```python
from build123d import *

# Parameters (mm, degrees)
ESQUISSE1_W             = 16
ESQUISSE1_H             = 28.1
ESQUISSE1_R             = 1.725
BOSS_EXTRU_1_DEPTH      = 8.6
ESQUISSE2_W             = 16
ESQUISSE2_H             = 14.6
ENL_V_MAT_EXTRU_2_DEPTH = 7
ENL_V_MAT_EXTRU_5_DEPTH = 16
ENL_V_MAT_EXTRU_6_DEPTH = 7
ENL_V_START             = -2
ENL_V_MAT_EXTRU_9_DEPTH = 18


with BuildPart() as part:
    # Esquisse1 → Boss.-Extru.1 (new body)
    with BuildSketch(Plane.XY):
        with Locations((-5.445538763, -0.094706778)):
            Rectangle(ESQUISSE1_W, ESQUISSE1_H)
        with Locations(Location((-5.445538763, 10.955293222, 0), (0, 0, 180))):
            Circle(ESQUISSE1_R, mode=Mode.SUBTRACT)
        with Locations(Location((-5.445538763, -11.144706778, 0), (0, 0, 180))):
            Circle(ESQUISSE1_R, mode=Mode.SUBTRACT)
    extrude(amount=BOSS_EXTRU_1_DEPTH)

    # Esquisse2 → Enlèv. mat.-Extru.2 (cut)
    with BuildSketch(Plane(origin=(0, 0, 0), x_dir=(-1, 0, 0), z_dir=(0, 0, -1))):
        with Locations((5.445538763, -0.344706778)):
            Rectangle(ESQUISSE2_W, ESQUISSE2_H)
    extrude(amount=-ENL_V_MAT_EXTRU_2_DEPTH, mode=Mode.SUBTRACT)

    # Esquisse4 → Enlèv. mat.-Extru.5 (cut)
    with BuildSketch(Plane(origin=(0, 0, 0), x_dir=(-1, 0, 0), z_dir=(0, 0, -1))):
        Polygon((8.103346265, -14.144706778), (13.445538763, -14.144706778), (13.445538763, -8.673372576), (6.156041758, -14.144706778), align=None)
    extrude(amount=-ENL_V_MAT_EXTRU_5_DEPTH, mode=Mode.SUBTRACT)

    # Esquisse5 → Enlèv. mat.-Extru.6 (cut)
    with BuildSketch(Plane(origin=(0, 0, 0), x_dir=(-1, 0, 0), z_dir=(0, 0, -1))):
        Polygon((-2.554461237, -7.644706778), (-2.554461237, -10.894706778), (10.445538763, -7.644706778), align=None)
        Polygon((13.445538763, 6.955293222), (13.445538763, 9.910651633), (3.808396856, 6.955293222), align=None)
    extrude(amount=-ENL_V_MAT_EXTRU_6_DEPTH, mode=Mode.SUBTRACT)

    # Esquisse6 → Enlèv. mat.-Extru.9 (cut)
    with BuildSketch(Plane(origin=(0, 0, 0), x_dir=(-1, 0, 0), z_dir=(0, 0, -1)).offset(ENL_V_START)):
        Polygon((-2.554461237, 13.955293222), (-2.554461237, 8.169439353), (4.78538363, 8.169439353), (13.445538763, 11.062366287), (13.445538763, 13.955293222), align=None)
        with BuildLine():
            Line((6.156041758, -14.144706778), (12.854526116, -9.116973515))
            Line((12.854526116, -9.116973515), (5.445538763, -9.419706778))
            ThreePointArc((5.445538763, -9.419706778), (6.66529796, -9.924947581), (7.170538763, -11.144706778))
            ThreePointArc((7.170538763, -11.144706778), (4.386718709, -12.506516271), (5.020364742, -9.472925677))
            Line((5.020364742, -9.472925677), (4.233785553, -9.571381546))
            Line((4.233785553, -9.571381546), (-2.554461237, -12.089845576))
            Line((-2.554461237, -12.089845576), (-2.554461237, -14.144706778))
            Line((-2.554461237, -14.144706778), (6.156041758, -14.144706778))
        make_face()
    extrude(amount=-ENL_V_MAT_EXTRU_9_DEPTH, mode=Mode.SUBTRACT)


solid = part.part
```
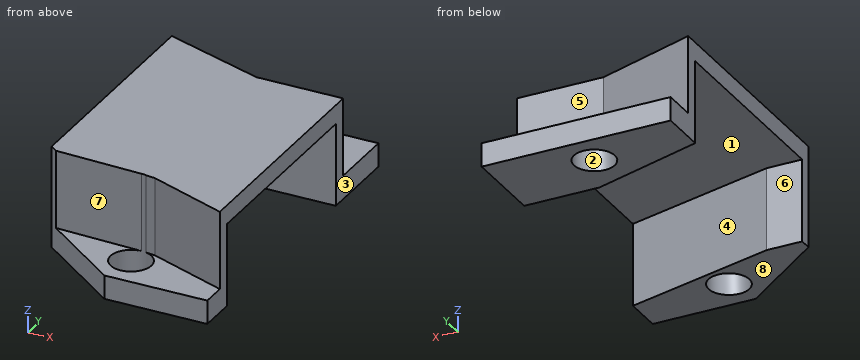
Geometry: final body of the model. Coordinates: model frame, mm. Face numbers are marked on the shaded views. A direction names the side the tool comes from. Coordinates: 2 decimals unless noted, no trailing zeros. Order: outer loops, then holes, each group sorted by start corner. A loop starts at its lowest first (then second) coordinate and runs counter-clockwise, first axis right, second up. Notation, with made-up numbers: M 40,75.25 L 79,75.25 A11 ccw 79,89.25 Z; hole C 27.5,-25.75 d10. An arc over 180 degrees is marked long. Answer in a Markdown table with one row per item. Add a question column.
Q1. Line query: L1, parallel to X at y = 11, z = 0.5; L2, parallel to Z at x = -7, y = -4.5; L3, parallel to Y at x = -11.25, z = 6.5. Output: solid intervals per line, ascending.
Q2. Section query A-A on z = 2.5. Return the cut outline in (x, y) (3 decimals).
Q3. Section query D-D on y = -8. Return the cut outline in (x, z), and give its area (3 significant figures).
Q4. Reachability of the marked faces 4, 5, 6, 7 and 8 from +Z, -Z, +X, -X, +Y, -Y: full face, straight path, thin tool, end or side. Return the list, or none.
Q5. Section query B-B on z = 7.5. Return the cut outline in (x, y) (3 decimals), and give its area (3 significant figures).
Q6. Section query C-C on y = 11.5. Return the cut outline in (x, z), and give its area (3 significant figures).
Q7. Mould query, pull axis X, two halves, no side actions, for the marked faces 1, 2 and 3. Classes: released by +X, released by -X, zero draft, split by the parting line, or undercut.
Q8. Contact query for flat-ended pins moving along their axis: P1, Ø2.5, axis at x = -4, y = -12, coming from the +Z side; P2, Ø8, axis at x = -7, y = 2, coming from the -Z side; P3, Ø1.5, axis at x = -11.5, z = 3, coming from the +Y side. Output: stop coordinate, or through.
Completed:
| question | item | result |
|---|---|---|
| 1 | L1 | x = -13.45 to -7.17, -3.72 to 2.55 |
| 1 | L2 | z = 7 to 8.6 |
| 1 | L3 | y = -9.18 to -7.64, 9.24 to 10.33 |
| 2 | outline | M -13.446,-8.673 L -12.855,-9.117 L -5.446,-9.42 A1.725 cw -5.02,-9.473 L -4.234,-9.571 L 2.554,-12.09 L 2.554,-10.895 L -10.446,-7.645 L -13.446,-7.645 Z; M -13.446,9.911 L -3.808,6.955 L 2.554,6.955 L 2.554,8.169 L -4.785,8.169 L -13.446,11.062 Z |
| 3 | outline | M -13.45,0 L -9.02,0 L -9.02,7 L 2.55,7 L 2.55,8.6 L -13.45,8.6 Z |
| 3 | area | 56.5 mm2 |
| 4 | face 4 | -Z, +X |
| 4 | face 5 | +Z, +X, +Y |
| 4 | face 6 | -Z, +X, -X |
| 4 | face 7 | +Z, -X, -Y |
| 4 | face 8 | -Z, +X, -X, +Y, -Y |
| 5 | outline | M -13.446,-8.673 L -12.855,-9.117 L -5.446,-9.42 A1.725 cw -5.02,-9.473 L -4.234,-9.571 L 2.554,-12.09 L 2.554,8.169 L -4.785,8.169 L -13.446,11.062 Z |
| 5 | area | 302 mm2 |
| 6 | outline | M -13.45,0 L -7.08,0 L -7.08,2 L -13.45,2 Z; M -3.81,0 L 2.55,0 L 2.55,2 L -3.81,2 Z |
| 6 | area | 25.5 mm2 |
| 7 | face 1 | zero draft |
| 7 | face 2 | undercut |
| 7 | face 3 | released by +X |
| 8 | P1 | stops at z = 2 |
| 8 | P2 | stops at z = 7 |
| 8 | P3 | stops at y = 10.66 |
